Verification items for the finished model (mm, model axes). A direction names the side the tool comes from. Round coordinates to 2 decimals unless told otherwise and drop trailing zeros. Loops run counter-clockwise (first coordinate to the right, second up) from the corner with the lowest first, then second, coordinate; pieces in that order, holes last. Notation, with made-up numbers: M 45,85 L 88,85 A3 ccw 88,90 Z; hole C -7,88.25 d4. An arc over 180 degrees is marked long. Answer as CSV lines item,"result".
```python
from build123d import *

# Parameters (mm, degrees)
PAD_DEPTH = 3


with BuildPart() as part:
    # Sketch → Pad (new body)
    with BuildSketch(Plane.XY):
        with BuildLine():
            Line((0, 126), (0, 1))
            ThreePointArc((0, 1), (0.292893, 0.292893), (1, 0))
            Line((1, 0), (14.748, 0))
            ThreePointArc((14.748, 0), (15.455107, 0.292893), (15.748, 1))
            Line((15.748, 12.7), (15.748, 1))
            ThreePointArc((22.352, 12.7), (19.05, 16.002), (15.748, 12.7))
            Line((22.352, 12.7), (22.352, 1))
            ThreePointArc((22.352, 1), (22.644893, 0.292893), (23.352, 0))
            Line((23.352, 0), (37.7002, 0))
            ThreePointArc((37.7002, 0), (38.407307, 0.292893), (38.7002, 1))
            Line((38.7002, 1), (38.7002, 24.9))
            ThreePointArc((39.7002, 25.9), (38.993093, 25.607107), (38.7002, 24.9))
            Line((39.7002, 25.9), (119.2001, 25.9))
            ThreePointArc((119.2001, 25.9), (119.907207, 26.192893), (120.2001, 26.9))
            Line((120.2001, 26.9), (120.2001, 126))
            ThreePointArc((120.2001, 126), (119.907207, 126.707107), (119.2001, 127))
            Line((119.2001, 127), (1, 127))
            ThreePointArc((1, 127), (0.292893, 126.707107), (0, 126))
        make_face()
    extrude(amount=PAD_DEPTH)


solid = part.part
```
1) Section check C-C (x = 103). Record the cut outline in (y, z), plus the area to 3 significant figures.
Here are the results:
outline,"M 25.9,0 L 127,0 L 127,3 L 25.9,3 Z"
area,"303 mm^2"
2) Go/stop test with a flat-tipped pin: pin 1 (1.5 mm diameter, centred on x = 85, y = 87.5, fed in from -Z). Record where the tip stops, or that it passes through.
Here are the results:
pin 1,"stops at z = 0"
3) Section check B-B (x = 19.05). Record the cut outline in (y, z), plus the area to 3 significant figures.
Here are the results:
outline,"M 16,0 L 127,0 L 127,3 L 16,3 Z"
area,"333 mm^2"
4) Set-up check for faces 1 (the flat face through (22.352, 7, 1)), 2 (the flat face through (61, 127, 1)), 3 (the flat face through (38.7, 13, 1)): record each of +Z, -Z, +X, -X, +Y, -Y from which the full face is reachable in a straight line by a thin tool's end or side.
Here are the results:
face 1,"+Z, -Z, -Y"
face 2,"+Z, -Z, +X, -X, +Y"
face 3,"+Z, -Z, +X, -Y"
5) Material ranges on probe 1 along X at (y, z) = (13, 2.7); probe 2 along X at (y, z) = (17, 2.35); probe 3 along X at (y, z) = (11, 2.05), recorded low to high.
Here are the results:
probe 1,"x = 0 to 15.76, 22.34 to 38.7"
probe 2,"x = 0 to 38.7"
probe 3,"x = 0 to 15.75, 22.35 to 38.7"
6) Section check A-A (z = 1). Record the cut outline in (x, y).
Here are the results:
outline,"M 0,1 A1 ccw 1,0 L 14.75,0 A1 ccw 15.75,1 L 15.75,12.7 A3.3 cw 22.35,12.7 L 22.35,1 A1 ccw 23.35,0 L 37.7,0 A1 ccw 38.7,1 L 38.7,24.9 A1 cw 39.7,25.9 L 119.2,25.9 A1 ccw 120.2,26.9 L 120.2,126 A1 ccw 119.2,127 L 1,127 A1 ccw 0,126 Z"
